Geometry check sheet. Reference: the model listing, model coordinates, mm. Face numbers are marked on the shaded views. A direction names the side the tool comes from. Round coordinates to 2 decimals unless told otherwise and drop trailing zeros. Order: outer loops, then holes, each group sorted by start corner. A loop starts at its lowest first (then second) coordinate and runs counter-clockwise, first axis right, second up.
(1) Go/stop test with flat-tipped pins: pin 1 (1.5 mm diameter, centred on x = 4.5, z = 2.5, fed in from -Y); pin 2 (1.5 mm diameter, centred on x = 5.5, z = 16.5, fed in from +Y). Record where each tip stops, or that it passes through.
(2) Sectioned sample at C-C (x = 5.5). Record the boundary of the cut face in (y, z).
(3) Set-up check for the marked faces 1 and 2: record each of +Z, -Z, +X, -X, +Y, -Y from which the full face is reachable in a straight line by a thin tool's end or side.
(4) Sectioned sample at B-B (z = 18). Record the boundary of the cut face in (x, y), plus the area to 3 significant figures.
(5) Material ranges on line 1 along Z through (x, y) = (1.25, 2.5); line 2 along Y through (x, z) = (4, 17); line 3 along X through (y, z) = (4, 20), recorded low to high.
(6) Sectioned sample at D-D (x = 1.75). Record the boundary of the cut face in (y, z), plus the area to 3 significant figures.
(7) Sectioned sample at A-A (x = 4). Record the boundary of the cut face in (y, z).
from build123d import *
from build123d.topology import SkipClean

# Parameters (mm, degrees)
SKETCH1_W               = 8
SKETCH1_H               = 6
BOSS_EXTRUDE1_DEPTH     = 15
SKETCH2_R               = 2
BOSS_EXTRUDE2_DEPTH     = 10
CUT_EXTRUDE1_DEPTH      = 27.925824036
CIRPATTERN1_DEPTH       = 15
CUT_EXTRUDE2_DEPTH      = 27.925824088
CUT_EXTRUDE2_DEPTH_BACK = 27.925824088
SKETCH4_W               = 8
SKETCH4_H               = 3


# Read off the part's stored shape, not the designer's step: CirPattern1
with BuildPart() as part:
    # Sketch1 → Boss-Extrude1 (new body)
    with BuildSketch(Plane.XY):
        with Locations((4, 3)):
            Rectangle(SKETCH1_W, SKETCH1_H)
    extrude(amount=BOSS_EXTRUDE1_DEPTH)

    # Sketch2 → Boss-Extrude2 (add)
    with BuildSketch(Plane.XY.offset(15)):
        with Locations((4, 3)):
            Circle(SKETCH2_R)
    extrude(amount=BOSS_EXTRUDE2_DEPTH)

    # Sketch3 → Cut-Extrude1 (cut, through all)
    with BuildSketch(Plane(origin=(0, 0, 0), x_dir=(-1, 0, 0), z_dir=(0, 0, -1))):
        with BuildLine():
            Line((-8, 0), (-6.5, 0))
            add(Edge.make_bspline(
                [(-6.5, 0), (-7.519049776, 1.013941068), (-7.906316023, 2.115854023), (-8, 3)],
                knots=[0, 0, 0, 0, 1, 1, 1, 1], degree=3))
            Line((-8, 3), (-8, 0))
        make_face()
    extrude(amount=-CUT_EXTRUDE1_DEPTH, mode=Mode.SUBTRACT)

    # CirPattern1 outline → CirPattern1 (cut)
    with BuildSketch(Plane.XY):
        with BuildLine():
            Line((0, 0), (1.5, 0))
            add(Edge.make_bspline(
                [(1.5, 0), (0.480950224, 1.013941068), (0.093683977, 2.115854023), (0, 3)],
                knots=[0, 0, 0, 0, 1, 1, 1, 1], degree=3))
            Line((0, 3), (0, 0))
        make_face()
    extrude(amount=CIRPATTERN1_DEPTH, mode=Mode.SUBTRACT)

    # Sketch4 → Cut-Extrude2 (cut, two sides: drawn at the far end of the back side and taken through both)
    with BuildSketch(Plane(origin=(0, 0, 0), x_dir=(-1, 0, 0), z_dir=(0, 0, -1)).offset(-CUT_EXTRUDE2_DEPTH_BACK)):
        with Locations((-4, 4.5)):
            Rectangle(SKETCH4_W, SKETCH4_H)
    extrude(amount=CUT_EXTRUDE2_DEPTH + CUT_EXTRUDE2_DEPTH_BACK, mode=Mode.SUBTRACT)

    # Mirror1: part across plane


with BuildPart() as part_1:
    with SkipClean():  # the faces are left unmerged after this step: merging them gives an invalid solid
        add(part.part)
        add(part.part.mirror(Plane(origin=(8, 3, 25), x_dir=(0, 0, 1), z_dir=(0, -1, 0))))


solid = part_1.part
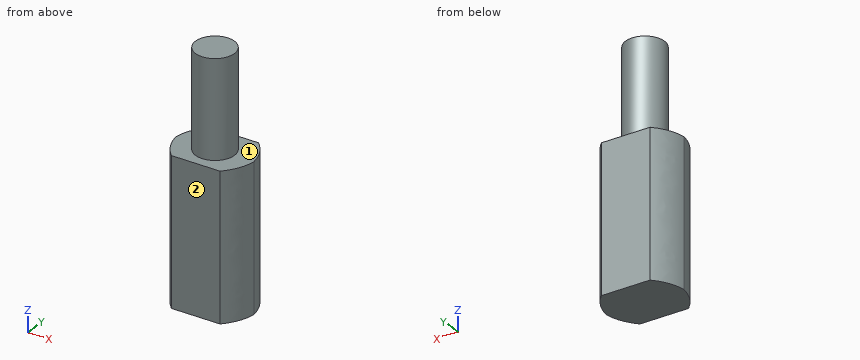
Answer below:
1. pin 1: stops at y = 0
1. pin 2: stops at y = 4.85
2. outline: (0, 0) - (6, 0) - (6, 15) - (4.32, 15) - (4.32, 25) - (1.68, 25) - (1.68, 15) - (0, 15) - close
3. face 1: +Z
3. face 2: +Z, -Z, +X, -X, -Y
4. outline: circle Ø4 at (4, 3)
4. area: 12.6 mm2
5. line 1: z = 0 to 15
5. line 2: y = 1 to 5
5. line 3: x = 2.27 to 5.73
6. outline: (0, 0) - (6, 0) - (6, 15) - (0, 15) - close
6. area: 90.0 mm2
7. outline: (0, 0) - (6, 0) - (6, 15) - (5, 15) - (5, 25) - (1, 25) - (1, 15) - (0, 15) - close
